from build123d import *

# Parameters (mm, degrees)
F0_R     = 75
F1_DEPTH = 12.7
F2_R     = 75
F2_R_2   = 59.252001
F3_DEPTH = 8.89
F4_R     = 10
F5_DEPTH = 25.4
F6_R     = 5.510782
F7_DEPTH = 25.4


with BuildPart() as f1:
    # F0 (on Front) → F1 (new body)
    with BuildSketch(Plane.XZ):
        Circle(F0_R)
    extrude(amount=F1_DEPTH)

    # F2 (on face) → F3 (join)
    with BuildSketch(Plane.XZ.offset(12.7)):
        Circle(F2_R)
        Circle(F2_R_2, mode=Mode.SUBTRACT)
    extrude(amount=F3_DEPTH)

    # F4 (on face) → F5 (cut)
    with BuildSketch(Plane.XZ.offset(12.7)):
        with Locations((-26.308898, 14.438962)):
            Circle(F4_R)
        with Locations((28.165994, 14.438962)):
            Circle(F4_R)
        with Locations((0, -33.466256)):
            Circle(F4_R)
    extrude(amount=-F5_DEPTH, mode=Mode.SUBTRACT)

    # F6 (on face) → F7 (cut)
    with BuildSketch(Plane.XZ.offset(21.59)):
        with Locations((0, 67.629345)):
            Circle(F6_R)
    extrude(amount=-F7_DEPTH, mode=Mode.SUBTRACT)


solid = f1.part
Source: CAD feature listing. Evaluate the final solid. Frame: model axes, mm. A direction names the side the tool comes from. Give positions to 0.01 mm unless a question says otherwise; leave off trailing zeros. Write each loop counter-clockwise with the first axis right and the second up, starting at its lowest first coordinate (ties: lowest second). Pieces come first, ordered by that corner, then holes. Notation, with made-up numbers: M -35.75,24 L 14.25,24 A16 ccw 14.25,30 Z; hole C -3,-34 d6. An arc over 180 degrees is marked long. Return JSON: item names as keys, results as strings. Group by question number.
1) Cut plane B-B, the plane x = -25.5. Output: boundary loops of the cut face in (y, z).
2) Material intervals for line 1 along Z through (x, y) = (0, -10.25); line 2 along Z through (x, y) = (0, -15.5); line 3 along Y through (x, z) = (-27, -39), sorted ascending. Write a range as [from, to].
3) Cut plane A-A, the plane x = 0. Output: boundary loops of the cut face in (y, z).
4) Cut plane C-C, the plane y = -7.5. Output: boundary loops of the cut face in (x, z).
5) Pin query (flat end, axial travel): P1, Ø3, axis at x = 30.5, z = 30.5, coming from the -Y side; P2, Ø10, axis at x = -17.5, y = -15, coming from the -Z side; P3, Ø10, axis at y = -3, z = -24, coming from the -X side. Return the tip coordinate at first contact, or that it passes through.
6) Set-up query: faces 1 (the face through (37.704, -6.439, 17.443)), 2 (the face through (-1, -12.7, 1)). Return all of +Z, -Z, +X, -X, +Y, -Y with unobstructed straight access to the full face (end or side cutting, diameter ignored); none if empty.
7) Pull-direction query (X, two-part tool) for faces 3 (the face through (-9.764, -10.644, 74.362)), 4 (the face through (-12.845, -17.083, -57.843)), 5 (the face through (-1.19, -10.95, 62.25)), 6 (the face through (-1, 0, 1)); classes: pulls with the +X half, pulls with the -X half, needs draft (parallel to the pull), parting line crosses it, or undercut.
8) Cut plane D-D, the plane z = 36.5. Output: boundary loops of the cut face in (x, y), plus the area to 3 significant figures.
Recorded:
{
 "1": {"outline": "M -21.59,-70.53 L 0,-70.53 L 0,4.47 L -12.7,4.47 L -12.7,-53.48 L -21.59,-53.48 Z; M -21.59,53.48 L -12.7,53.48 L -12.7,24.41 L 0,24.41 L 0,70.53 L -21.59,70.53 Z"},
 "2": {"line 1": "z = [-75, -43.47], [-23.47, 62.12], [73.14, 75]", "line 2": "z = [-75, -59.25], [59.25, 62.12], [73.14, 75]", "line 3": "y = [-12.7, 0]"},
 "3": {"outline": "M -21.59,-75 L 0,-75 L 0,-43.47 L -12.7,-43.47 L -12.7,-59.25 L -21.59,-59.25 Z; M -21.59,59.25 L -12.7,59.25 L -12.7,-23.47 L 0,-23.47 L 0,62.12 L -21.59,62.12 Z; M -21.59,73.14 L 0,73.14 L 0,75 L -21.59,75 Z"},
 "4": {"outline": "C 0,0 d150; hole C -26.31,14.44 d20; hole C 0,-33.47 d20; hole C 0,67.63 d11.02; hole C 28.17,14.44 d20"},
 "5": {"P1": "stops at y = -12.7", "P2": "stops at z = -73.95", "P3": "stops at x = -72.55"},
 "6": {"face 1": "+Y, -Y", "face 2": "-Y"},
 "7": {"face 3": "parting line crosses it", "face 4": "undercut", "face 5": "undercut", "face 6": "needs draft"},
 "8": {"outline": "M -65.52,-21.59 L -46.67,-21.59 L -46.67,-12.7 L 46.67,-12.7 L 46.67,-21.59 L 65.52,-21.59 L 65.52,0 L -65.52,0 Z", "area": "2,000 mm²"}
}
